```python
from build123d import *

# Parameters (mm, degrees)
SKETCH2_R           = 2.0828
SKETCH2_R_2         = 20.32
BOSS_EXTRUDE1_DEPTH = 3.175


with BuildPart() as part:
    # Sketch2 → Boss-Extrude1 (new body)
    with BuildSketch(Plane(origin=(0, 0, 0), x_dir=(1, 0, 0), z_dir=(0, 1, 0))):
        with BuildLine():
            Line((15.875, 0), (15.875, 12.7))
            Line((15.875, 12.7), (12.7, 12.7))
            Line((12.7, 12.7), (12.7, 25.4))
            Line((12.7, 25.4), (15.875, 25.4))
            Line((15.875, 25.4), (15.875, 38.1))
            Line((15.875, 38.1), (12.7, 38.1))
            Line((12.7, 38.1), (12.7, 50.8))
            Line((12.7, 50.8), (15.875, 50.8))
            Line((15.875, 50.8), (15.875, 63.5))
            Line((15.875, 63.5), (12.7, 63.5))
            Line((12.7, 63.5), (12.7, 76.2))
            Line((12.7, 76.2), (15.875, 76.2))
            Line((15.875, 76.2), (15.875, 88.9))
            Line((15.875, 88.9), (12.7, 88.9))
            Line((12.7, 88.9), (12.7, 101.6))
            Line((12.7, 101.6), (15.875, 101.6))
            Line((15.875, 101.6), (32.385, 101.6))
            ThreePointArc((32.385, 101.6), (34.925, 99.06), (37.465, 101.6))
            Line((37.465, 101.6), (121.285, 101.6))
            ThreePointArc((121.285, 101.6), (123.825, 99.06), (126.365, 101.6))
            Line((126.365, 101.6), (142.875, 101.6))
            Line((142.875, 101.6), (142.875, 88.9))
            Line((142.875, 88.9), (146.05, 88.9))
            Line((146.05, 88.9), (146.05, 76.2))
            Line((146.05, 76.2), (142.875, 76.2))
            Line((142.875, 76.2), (142.875, 63.5))
            Line((142.875, 63.5), (146.05, 63.5))
            Line((146.05, 63.5), (146.05, 50.8))
            Line((146.05, 50.8), (142.875, 50.8))
            Line((142.875, 50.8), (142.875, 38.1))
            Line((142.875, 38.1), (146.05, 38.1))
            Line((146.05, 38.1), (146.05, 25.4))
            Line((146.05, 25.4), (142.875, 25.4))
            Line((142.875, 25.4), (142.875, 12.7))
            Line((142.875, 12.7), (146.05, 12.7))
            Line((146.05, 12.7), (146.05, 0))
            Line((146.05, 0), (15.875, 0))
        make_face()
        with Locations(Location((41.275, 57.15, 0), (0, 0, 270))):
            Circle(SKETCH2_R, mode=Mode.SUBTRACT)
        with Locations(Location((136.525, 6.35, 0), (0, 0, 90))):
            Circle(SKETCH2_R, mode=Mode.SUBTRACT)
        with Locations(Location((79.375, 29.972, 0), (0, 0, 270))):
            Circle(SKETCH2_R_2, mode=Mode.SUBTRACT)
        with Locations(Location((22.225, 6.35, 0), (0, 0, 270))):
            Circle(SKETCH2_R, mode=Mode.SUBTRACT)
        with Locations(Location((117.475, 57.15, 0), (0, 0, 90))):
            Circle(SKETCH2_R, mode=Mode.SUBTRACT)
        with Locations(Location((22.225, 95.25, 0), (0, 0, 90))):
            Circle(SKETCH2_R, mode=Mode.SUBTRACT)
        with Locations(Location((136.525, 95.25, 0), (0, 0, 270))):
            Circle(SKETCH2_R, mode=Mode.SUBTRACT)
    extrude(amount=BOSS_EXTRUDE1_DEPTH)


solid = part.part
```
Part model, mm, in its own coordinate system. A direction names the side the tool comes from. Round coordinates to 2 decimals unless told otherwise and drop trailing zeros. Loops run counter-clockwise (first coordinate to the right, second up) from the corner with the lowest first, then second, coordinate; pieces in that order, holes last.
Item 1: 3-axis set-ups, long thin cutter, end or side, ignore diameter. For faces 4 (the face through (142.875, 2, -19)), 5 (the face through (146.05, 2, -6)), 6 (the face through (15.875, 2, -57)): which of +Z, -Z, +X, -X, +Y, -Y reach the whole face in a straight line?
Item 2: Cut at C-C, the plane x = 75. Give the cut face in (y, z) (3 decimals).
Item 3: Drill centre lines: line 1 (X direction, y = 1.8, z = -6.35) (3 decimals); line 2 (X direction, y = 1.35, z = -95.25) (3 decimals); line 3 (X direction, y = 1.45, z = -71) (3 decimals). Where is each one in solid material? Low to high.
Item 4: Cut at A-A, the plane z = -6.35. Give the cut face in (x, y) (3 decimals), then the cut area to 3 significant figures.
Item 5: Cut at B-B, the plane z = -35. Give the cut face in (x, y) (3 decimals).
Item 6: Mould opens along X. For faces 1 (the face through (61.348, 1.565, -20.596)), 2 (the face through (144, 2, -88.9)), 3 (the face through (142.875, 2, -95)) say: +X half, -X half, draft (parallel to the pull), parting line (faces both ways), or undercut.
Item 7: Cut at D-D, the plane y = 1.25. State how many separate pieces and enclosed holes the cut face has, then the cut area to 3 significant figures.
Item 8: Drop flat-ended pins along their axis: P1, Ø1.6, axis at x = 145, y = 1, coming from the +Z side; P2, Ø1.6, axis at x = 144, y = 1.5, coming from the -Z side; P3, Ø1.6, axis at y = 2, z = -9, coming from the -X side (3 decimals); P4, Ø1, axis at x = 13.5, y = 1, coming from the +Z side. Give the stop position or say it passes through.
A:
1. face 4: +X, +Y, -Y
1. face 5: +Z, -Z, +X, +Y, -Y
1. face 6: -X, +Y, -Y
2. outline: (0, -101.6) - (3.175, -101.6) - (3.175, -49.815) - (0, -49.815) - close; (0, -10.129) - (3.175, -10.129) - (3.175, 0) - (0, 0) - close
3. line 1: x = 15.875 to 20.142, 24.308 to 134.442, 138.608 to 146.05
3. line 2: x = 12.7 to 20.142, 24.308 to 134.442, 138.608 to 142.875
3. line 3: x = 12.7 to 142.875
4. outline: (15.875, 0) - (20.142, 0) - (20.142, 3.175) - (15.875, 3.175) - close; (24.308, 0) - (134.442, 0) - (134.442, 3.175) - (24.308, 3.175) - close; (138.608, 0) - (146.05, 0) - (146.05, 3.175) - (138.608, 3.175) - close
4. area: 387 mm2
5. outline: (15.875, 0) - (59.687, 0) - (59.687, 3.175) - (15.875, 3.175) - close; (99.063, 0) - (146.05, 0) - (146.05, 3.175) - (99.063, 3.175) - close
6. face 1: undercut
6. face 2: draft
6. face 3: +X half
7. separate pieces: 1
7. enclosed holes: 7
7. area: 11,800 mm2
8. P1: stops at z = 0
8. P2: stops at z = -88.9
8. P3: stops at x = 15.875
8. P4: stops at z = -12.7
